Print and shaded views of the part. All mm, measured from the part's lowest x, y and z. A direction names the side the tool comes from. Coordinates: 2 decimals unless noted, no trailing zeros. Order: outer loops, then holes, each group sorted by start corner. A loop starts at its lowest first (then second) coordinate and runs counter-clockwise, first axis right, second up. Notation, with made-up numbers: (65, 8) -> (97, 8) arc R17 ccw to (97, 36) -> close; hole circle Ø6 at (26, 78.5). An arc over 180 degrees is marked (long way). Return JSON: item names as keys, results as strings. Group by question number.
1) Cut at C-C (x = 56.5). Write the cut outline in (y, z) (1 decimal).
2) Cut at D-D (y = 16). Write the cut outline in (x, z) (1 decimal), and give its area (3 significant figures).
3) Which spindle directions (+Z, -Z, +X, -X, +Y, -Y) get a long thin tool onto all of the face, cutting with end or side? Do the marked faces 1 and 2. Say none if no direction does.
4) Pull direction X, two halves, no side cores. Call the marked faces 3, 4 and 5: +X half, -X half, draft (parallel to the pull), parting line (faces both ways), or undercut.
5) Probe line 1 (Y direction, x = 4, z = 3.25); line 2 (Z direction, x = 7.5, y = 26.65); line 3 (X direction, y = 32.3, z = 10). List the from-to ranges inside material, lowest first.
6) Cut at B-B (y = 25.5). State how many separate pieces and enclosed holes the cut face has, and give its area (3 significant figures).
7) Flat gauge pins, fed straight in: pin 1 (4 mm diameter, centred on x = 7.5, z = 10, fed in from +Y); pin 2 (1 mm diameter, centred on y = 11.5, z = 15, fed in from -X); pin 3 (12 mm diameter, centred on y = 47, z = 17.5, fed in from +X); pin 4 (6 mm diameter, centred on x = 8.5, z = 6, fed in from +Y). Where does each tip first touch, or does it go through?
8) Cut at A-A (z = 10). Write the cut outline in (x, y).
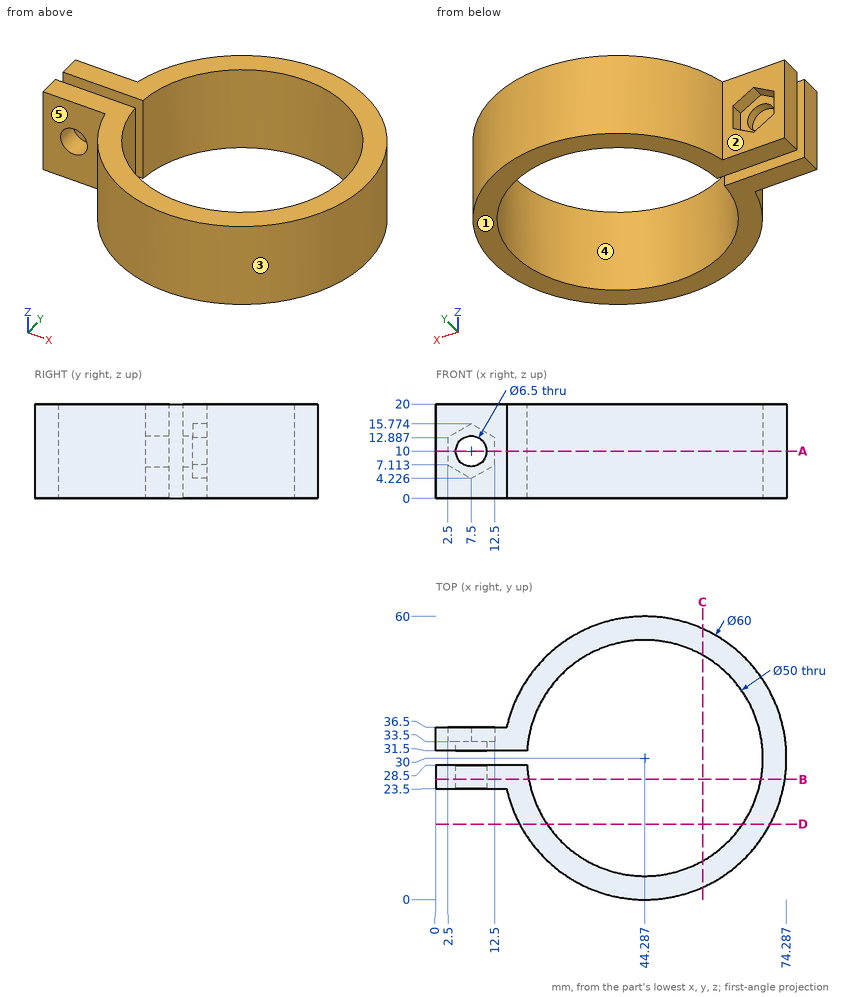
Answers below:
{
 "1": {"outline": "(2.6, 0) -> (8.2, 0) -> (8.2, 20) -> (2.6, 20) -> close; (51.8, 0) -> (57.4, 0) -> (57.4, 20) -> (51.8, 20) -> close"},
 "2": {"outline": "(17.8, 0) -> (23.6, 0) -> (23.6, 20) -> (17.8, 20) -> close; (65, 0) -> (70.8, 0) -> (70.8, 20) -> (65, 20) -> close", "area": "233 mm^2"},
 "3": {"face 1": "-Z, +X, -X, +Y, -Y", "face 2": "+Z, -Z, -X, +Y"},
 "4": {"face 3": "parting line", "face 4": "undercut", "face 5": "draft"},
 "5": {"line 1": "y = 23.5 to 28.5, 31.5 to 36.5", "line 2": "z = 0 to 6.75, 13.25 to 20", "line 3": "x = 0 to 4.25, 10.75 to 19.39, 69.18 to 74.2"},
 "6": {"separate pieces": "2", "enclosed holes": "1", "area": "462 mm^2"},
 "7": {"pin 1": "passes through", "pin 2": "stops at x = 20.29", "pin 3": "stops at x = 72.2", "pin 4": "stops at y = 36.5"},
 "8": {"outline": "(0, 23.5) -> (4.25, 23.5) -> (4.25, 28.5) -> (0, 28.5) -> close; (0, 31.5) -> (4.25, 31.5) -> (4.25, 33.5) -> (2.5, 33.5) -> (2.5, 36.5) -> (0, 36.5) -> close; (10.75, 23.5) -> (15, 23.5) arc R30 ccw (long way) to (15, 36.5) -> (12.5, 36.5) -> (12.5, 33.5) -> (10.75, 33.5) -> (10.75, 31.5) -> (19.33, 31.5) arc R25 cw (long way) to (19.33, 28.5) -> (10.75, 28.5) -> close"}
}
